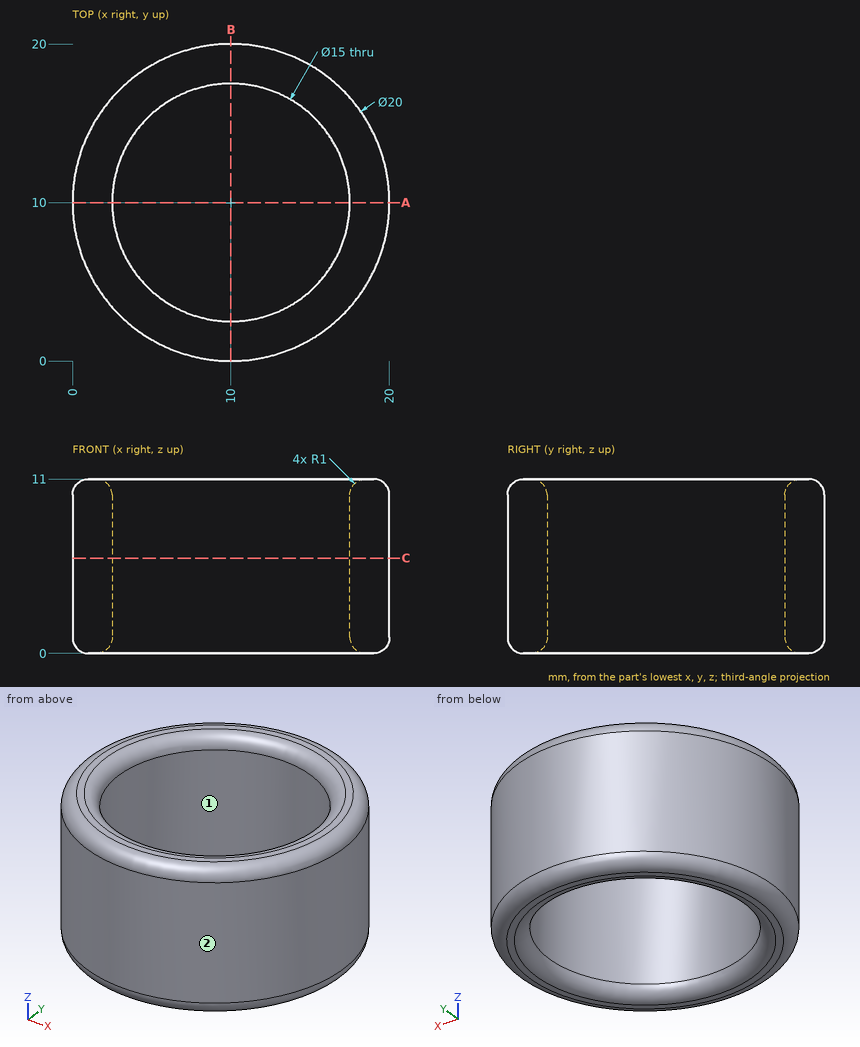
Design review of the part shown in the three views and the two pictorial views. Dimensions are in mm from the part's minimum x, y and z. Give positions to 0.01 mm unless a question says otherwise; leave off trailing zeros. Loops run counter-clockwise (first coordinate to the right, second up) from the corner with the lowest first, then second, coordinate; pieces in that order, holes last. Notation, with made-up numbers: (-22.5, 58) -> (-2.5, 58) arc R30 cw to (-2.5, 97) -> close; hole circle Ø2 at (-24.5, 13.25). An arc over 180 degrees is marked (long way). Answer as a JSON object with one key per item and string values. Group by question number.
Q1. Draft analysis for pull direction Y (two halves, no side actions). For the marked faces 1 and 2, state which applies: pulls with the +Y half, pulls with the -Y half, needs draft (parallel to the pull), parting line crosses it, or undercut.
Q2. Wall thickness on line 1 along Y through (x, z) = (10, 4.75); line 2 along Y through (x, z) = (12.25, 5); line 3 along X through (y, z) = (8, 6): over which ranges is each line inside the solid? List them lowest first.
Q3. Insertion check: pin 1 (8 mm diameter, centred on x = 5.5, y = 16, fed in from +Z); pin 2 (1 mm diameter, centred on y = 9, z = 6.5, fed in from +X); pin 3 (1 mm diameter, centred on x = 15, z = 6, fed in from -Y). Each pin has a flat end and moves straight along its axis. Give the tip position at first contact, or say it passes through.
Q4. Take a section at C-C (z = 6). Write out the cut boundary in (x, y), plus the area to 3 significant figures.
Q5. Take a section at A-A (y = 10). Write out the cut boundary in (x, z).
Answer below:
{
 "1": {"face 1": "undercut", "face 2": "parting line crosses it"},
 "2": {"line 1": "y = 0 to 2.5, 17.5 to 20", "line 2": "y = 0.26 to 2.85, 17.15 to 19.74", "line 3": "x = 0.2 to 2.77, 17.23 to 19.8"},
 "3": {"pin 1": "stops at z = 11", "pin 2": "stops at x = 19.99", "pin 3": "stops at y = 1.07"},
 "4": {"outline": "circle Ø20 at (10, 10); hole circle Ø15 at (10, 10)", "area": "137 mm2"},
 "5": {"outline": "(0, 1) arc R1 ccw to (1, 0) -> (1.5, 0) arc R1 ccw to (2.5, 1) -> (2.5, 10) arc R1 ccw to (1.5, 11) -> (1, 11) arc R1 ccw to (0, 10) -> close; (17.5, 1) arc R1 ccw to (18.5, 0) -> (19, 0) arc R1 ccw to (20, 1) -> (20, 10) arc R1 ccw to (19, 11) -> (18.5, 11) arc R1 ccw to (17.5, 10) -> close"}
}
